```python
from build123d import *

# Parameters (mm, degrees)
SKETCH2_W           = 50
SKETCH2_H           = 25
BOSS_EXTRUDE2_DEPTH = 5
CUT_EXTRUDE1_DEPTH  = 5


with BuildPart() as part:
    # Sketch2 → Boss-Extrude2 (new body)
    with BuildSketch(Plane.XY):
        Rectangle(SKETCH2_W, SKETCH2_H)
    extrude(amount=BOSS_EXTRUDE2_DEPTH)

    # Sketch6 → Cut-Extrude1 (cut)
    with BuildSketch(Plane.XY):
        with BuildLine():
            Line((-5, 12.5), (5, 12.5))
            ThreePointArc((5, 12.5), (0, 7.5), (-5, 12.5))
        make_face()
    extrude(amount=CUT_EXTRUDE1_DEPTH, mode=Mode.SUBTRACT)


solid = part.part
```
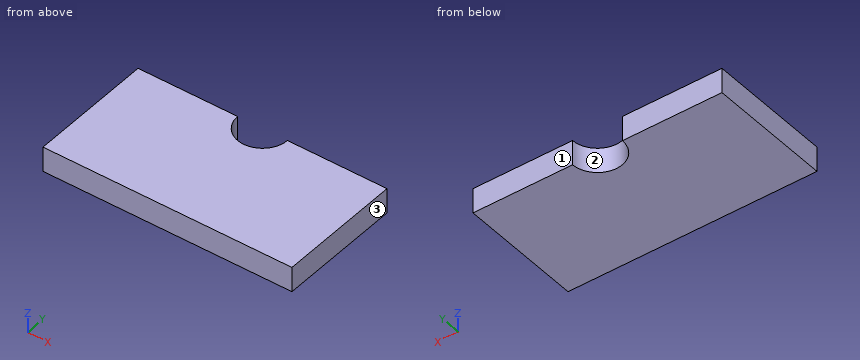
CAD build for the part. Positions are in the model's coordinates, mm. Face numbers are marked on the shaded views. Round coordinates to 2 decimals unless told otherwise and drop trailing zeros. Order: outer loops, then holes, each group sorted by start corner. A loop starts at its lowest first (then second) coordinate and runs counter-clockwise, first axis right, second up. Notation, with made-up numbers: (-33, 10) -> (25, 10) arc R14 ccw to (25, 30) -> close; hole circle Ø11 at (22.5, -21). An arc over 180 degrees is marked (long way). Write item = value, one per line.
(1) Cut at A-A (y = 9.5). Write the cut outline in (x, z).
Answers follow:
outline = (-25, 0) -> (-4, 0) -> (-4, 5) -> (-25, 5) -> close; (4, 0) -> (25, 0) -> (25, 5) -> (4, 5) -> close
(2) Cut at B-B (z = 3.4). Write the cut outline in (x, y).
Answers follow:
outline = (-25, -12.5) -> (25, -12.5) -> (25, 12.5) -> (5, 12.5) arc R5 cw to (-5, 12.5) -> (-25, 12.5) -> close
(3) Pull direction X, two halves, no side cores. Call the marked faces 1, 2 and 3: +X half, -X half, draft (parallel to the pull), parting line (faces both ways), or undercut.
Answers follow:
face_1 = draft
face_2 = undercut
face_3 = +X half
(4) Drill centre lines: L1, parallel to X at y = 11, z = 1.2; L2, parallel to X at y = 9.5, z = 2; L3, parallel to Y at x = -1, z = 4.8. Where is each one in solid material? Low to high.
Answers follow:
L1 = -25 to -4.77, 4.77 to 25
L2 = -25 to -4, 4 to 25
L3 = -12.5 to 7.6
(5) Cut at C-C (x = 0). Write the cut outline in (y, z).
Answers follow:
outline = (-12.5, 0) -> (7.5, 0) -> (7.5, 5) -> (-12.5, 5) -> close
